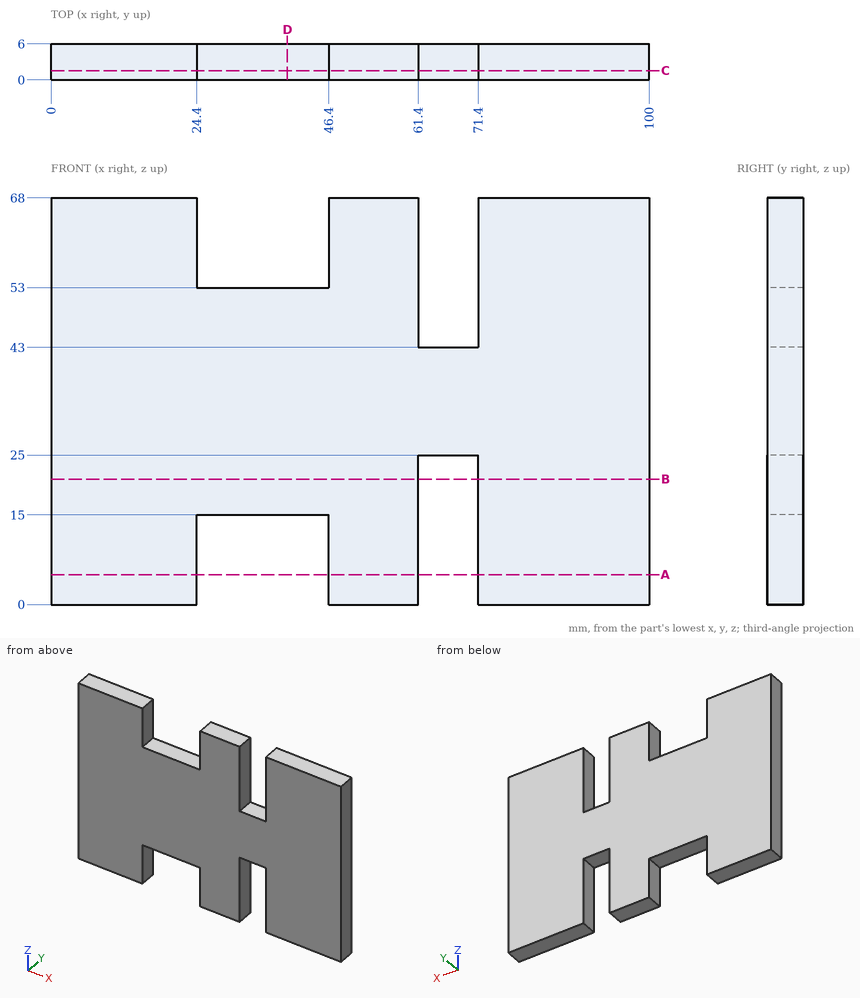
Geometry: see drawing. Coordinates: mm, zero at the bounding-box minimum. Round coordinates to 2 decimals unless told otherwise and drop trailing zeros. Write each loop counter-clockwise with the first axis right and the second up, starting at its lowest first coordinate (ties: lowest second). Pieces come first, ordered by that corner, then holes.
1) Cut plane D-D (x = 39.5). Return the cut outline in (y, z).
2) Cut plane C-C (y = 1.55). Return the cut outline in (x, z).
3) Contact query for flat-ended pins moving along their axis: P1, Ø2, axis at x = 63.5, y = 5.5, coming from the -Z side; P2, Ø3, axis at x = 40, y = 2, coming from the +Z side. Output: stop coordinate, or through.
4) Cut plane A-A (z = 5). Return the cut outline in (x, y).
5) Cut plane B-B (z = 21). Return the cut outline in (x, y), then the cut area to 3 significant figures.
6) Ray query, L1, parallel to X at y = 4.15, z = 54; L2, parallel to Z at x = 71, y = 2.7; L3, parallel to X at y = 4.25, z = 23. Return the intervals inside material, ascending.
Geometry says:
1. outline: (0, 15) - (6, 15) - (6, 53) - (0, 53) - close
2. outline: (0, 0) - (24.4, 0) - (24.4, 15) - (46.4, 15) - (46.4, 0) - (61.4, 0) - (61.4, 25) - (71.4, 25) - (71.4, 0) - (100, 0) - (100, 68) - (71.4, 68) - (71.4, 43) - (61.4, 43) - (61.4, 68) - (46.4, 68) - (46.4, 53) - (24.4, 53) - (24.4, 68) - (0, 68) - close
3. P1: stops at z = 25
3. P2: stops at z = 53
4. outline: (0, 0) - (24.4, 0) - (24.4, 6) - (0, 6) - close; (46.4, 0) - (61.4, 0) - (61.4, 6) - (46.4, 6) - close; (71.4, 0) - (100, 0) - (100, 6) - (71.4, 6) - close
5. outline: (0, 0) - (61.4, 0) - (61.4, 6) - (0, 6) - close; (71.4, 0) - (100, 0) - (100, 6) - (71.4, 6) - close
5. area: 540 mm2
6. L1: x = 0 to 24.4, 46.4 to 61.4, 71.4 to 100
6. L2: z = 25 to 43
6. L3: x = 0 to 61.4, 71.4 to 100
